Geometry: final body of the model. Coordinates: model frame, mm. A direction names the side the tool comes from. Give positions to 0.01 mm unless a question says otherwise; leave off trailing zeros. Write each loop counter-clockwise with the first axis right and the second up, starting at its lowest first coordinate (ties: lowest second). Pieces come first, ordered by that corner, then holes. Notation, with made-up numbers: (-6, -23) - (38, -23) arc R19 ccw to (38, -10) - close; hole circle Ø11 at (15, 22.25). An arc over 180 degrees is marked (long way). Use CSV: the item, a comma, the result in double quotes. Start each with the question number.
(1) Section A-A on z = 0.9. Output: boundary loops of the cut face in (x, y).
(2) Draft query along X for faces 1 (the cylindrical face through (-6, 0, 1)), 2 (the flat face through (142, 0, 6)), 3 (the cylindrical face through (12.11, -3.1, 2.49)). Return one class per face: released by +X, released by -X, zero draft, split by the parting line, or undercut.
(3) Section B-B on x = 28. Output: boundary loops of the cut face in (y, z), and give its area (3 significant figures).
(4) Line query: probe 1 along Y at (x, z) = (0, 1.9); probe 2 along X at (y, z) = (1, 0.6); probe 3 along Z at (x, y) = (23, 2.75). Output: solid intervals per line, ascending. Write a range as [from, to].
(5) First-contact query: pin 1 Ø4 at (x, y) = (141.5, -1) entering from -Z; pin 2 Ø3.5 at (x, y) = (34.5, 2) entering from +Z; pin 3 Ø1.5 at (y, z) = (-4.5, 1) entering from -X. Flat tips, straight axial feed; report the tip coordinate or a pass-through.
(6) Reachability of faces 4 (the cylindrical face through (12.11, 3.1, 2.49)), 5 (the flat face through (70, 6, 1)), 6 (the cylindrical face through (146.315, 1.201, 1.479)) from +Z, -Z, +X, -X, +Y, -Y: full face, straight path, thin tool, end or side. Return the list, or none.
(7) Section C-C on x = 10. Output: boundary loops of the cut face in (y, z).
from build123d import *

# Parameters (mm, degrees)
SKETCH1_R           = 4
BOSS_EXTRUDE1_DEPTH = 3
SKETCH3_R           = 5
BOSS_EXTRUDE2_DEPTH = 3
SKETCH4_W           = 120
SKETCH4_H           = 8
CUT_EXTRUDE1_DEPTH  = 1
FILLET1_R           = 3


with BuildPart() as part:
    # Sketch1 → Boss-Extrude1 (new body)
    with BuildSketch(Plane.XY):
        with BuildLine():
            Line((0, 6), (142.5, 6))
            ThreePointArc((142.5, 6), (148.5, 0), (142.5, -6))
            Line((142.5, -6), (0, -6))
            ThreePointArc((0, -6), (-6, 0), (0, 6))
        make_face()
        Circle(SKETCH1_R, mode=Mode.SUBTRACT)
        with Locations((142.5, 0)):
            Circle(SKETCH1_R, mode=Mode.SUBTRACT)
    extrude(amount=BOSS_EXTRUDE1_DEPTH)

    # Sketch3 → Boss-Extrude2 (add)
    with BuildSketch(Plane.XY.offset(3)):
        with Locations((142.5, 0)):
            Circle(SKETCH3_R)
    extrude(amount=BOSS_EXTRUDE2_DEPTH)

    # Sketch4 → Cut-Extrude1 (cut)
    with BuildSketch(Plane.XY.offset(3)):
        with Locations((71.25, 0)):
            Rectangle(SKETCH4_W, SKETCH4_H)
    extrude(amount=-CUT_EXTRUDE1_DEPTH, mode=Mode.SUBTRACT)

    # Fillet1
    fillet1_edges = [part.edges().sort_by_distance(p)[0] for p in [
        (131.25, 4, 2.5),
        (131.25, -4, 2.5),
        (11.25, -4, 2.5),
        (11.25, 4, 2.5),
    ]]
    fillet(fillet1_edges, radius=FILLET1_R)


solid = part.part
Check values:
1,outline,"(0, -6) - (142.5, -6) arc R6 ccw to (142.5, 6) - (0, 6) arc R6 ccw to start; hole circle Ø8 at (0, 0); hole circle Ø8 at (142.5, 0)"
2,face 1,"released by -X"
2,face 2,"zero draft"
2,face 3,"undercut"
3,outline,"(-6, 0) - (6, 0) - (6, 3) - (4, 3) - (4, 2) - (-4, 2) - (-4, 3) - (-6, 3) - close"
3,area,"28.0 mm²"
4,probe 1,"y = [-6, -4], [4, 6]"
4,probe 2,"x = [-5.92, -3.87], [3.87, 138.63], [146.37, 148.42]"
4,probe 3,"z = [0, 2]"
5,pin 1,"stops at z = 3"
5,pin 2,"stops at z = 2"
5,pin 3,"stops at x = -4.68"
6,face 4,"+Z"
6,face 5,"+Z, -Z, +X, -X, +Y"
6,face 6,"-Z"
7,outline,"(-6, 0) - (6, 0) - (6, 3) - (-6, 3) - close"
